```python
from build123d import *

# Parameters (mm, degrees)
EXTRUDE_1_DEPTH     = 8
SKETCH_3_R          = 16.5
CUT_EXTRUDE_1_DEPTH = 8
SKETCH_2_R          = 4
CUT_EXTRUDE_2_DEPTH = 60
SKETCH_4_R          = 4
CUT_EXTRUDE_3_DEPTH = 60
SKETCH_5_R          = 4
CUT_EXTRUDE_4_DEPTH = 60
SKETCH_6_R          = 4
CUT_EXTRUDE_5_DEPTH = 60
CUT_EXTRUDE_6_DEPTH = 1
SKETCH_8_R          = 2
CUT_EXTRUDE_8_DEPTH = 9


with BuildPart() as part:
    # 草图1 → 凸台-拉伸1 (new body)
    with BuildSketch(Plane(origin=(0, 0, 0), x_dir=(1, 0, 0), z_dir=(0, 1, 0))):
        Polygon((-40, 55), (-50, 45), (-50, -45), (-40, -55), (40, -55), (50, -45), (50, 45), (40, 55), align=None)
    extrude(amount=EXTRUDE_1_DEPTH)

    # 草图3 → 切除-拉伸1 (cut)
    with BuildSketch(Plane(origin=(0, 8, 0), x_dir=(1, 0, 0), z_dir=(0, 1, 0))):
        with Locations(Location((0, 0, 0), (0, 0, 270))):
            Circle(SKETCH_3_R)
    extrude(amount=-CUT_EXTRUDE_1_DEPTH, mode=Mode.SUBTRACT)

    # 草图2 → 切除-拉伸2 (cut)
    with BuildSketch(Plane(origin=(47.5, 0, 47.5), x_dir=(0.7071067811865483, 0, -0.7071067811865468), z_dir=(0.7071067811865468, 0, 0.7071067811865483))):
        with Locations((-3.535533906, 6)):
            Circle(SKETCH_2_R)
    extrude(amount=-CUT_EXTRUDE_2_DEPTH, mode=Mode.SUBTRACT)

    # 草图4 → 切除-拉伸3 (cut)
    with BuildSketch(Plane(origin=(-47.5, 0, 47.5), x_dir=(0.7071067811865475, 0, 0.7071067811865477), z_dir=(-0.7071067811865477, 0, 0.7071067811865475))):
        with Locations((3.535533906, 6)):
            Circle(SKETCH_4_R)
    extrude(amount=-CUT_EXTRUDE_3_DEPTH, mode=Mode.SUBTRACT)

    # 草图5 → 切除-拉伸4 (cut)
    with BuildSketch(Plane(origin=(-47.5, 0, -47.5), x_dir=(-0.7071067811865477, 0, 0.7071067811865475), z_dir=(-0.7071067811865475, 0, -0.7071067811865477))):
        with Locations((-3.535533906, 6)):
            Circle(SKETCH_5_R)
    extrude(amount=-CUT_EXTRUDE_4_DEPTH, mode=Mode.SUBTRACT)

    # 草图6 → 切除-拉伸5 (cut)
    with BuildSketch(Plane(origin=(47.5, 0, -47.5), x_dir=(-0.7071067811865475, 0, -0.7071067811865477), z_dir=(0.7071067811865477, 0, -0.7071067811865475))):
        with Locations((3.535533906, 6)):
            Circle(SKETCH_6_R)
    extrude(amount=-CUT_EXTRUDE_5_DEPTH, mode=Mode.SUBTRACT)

    # 草图7 → 切除-拉伸6 (cut)
    with BuildSketch(Plane(origin=(0, 8, 0), x_dir=(1, 0, 0), z_dir=(0, 1, 0))):
        Polygon((0, 47.334494774), (-7.385524007, 39.948970766), (7.385524007, 39.948970766), align=None)
    extrude(amount=-CUT_EXTRUDE_6_DEPTH, mode=Mode.SUBTRACT)

    # 草图8 → 切除-拉伸8 (cut)
    with BuildSketch(Plane(origin=(0, 8, 0), x_dir=(1, 0, 0), z_dir=(0, 1, 0))):
        with Locations(Location((-32.511046196, 47.511046196, 0), (0, 0, 270))):
            Circle(SKETCH_8_R)
        with Locations(Location((-42.504921706, 37.504921706, 0), (0, 0, 270))):
            Circle(SKETCH_8_R)
        with Locations(Location((-16.594623736, 31.594623736, 0), (0, 0, 270))):
            Circle(SKETCH_8_R)
        with Locations(Location((-26.594623736, 21.594623736, 0), (0, 0, 270))):
            Circle(SKETCH_8_R)
        with Locations(Location((16.828543077, 31.828543077, 0), (0, 0, 270))):
            Circle(SKETCH_8_R)
        with Locations(Location((32.511046196, 47.511046196, 0), (0, 0, 270))):
            Circle(SKETCH_8_R)
        with Locations(Location((42.504921706, 37.504921706, 0), (0, 0, 270))):
            Circle(SKETCH_8_R)
        with Locations(Location((26.57676385, 21.57676385, 0), (0, 0, 270))):
            Circle(SKETCH_8_R)
        with Locations(Location((-26.63034351, -21.63034351, 0), (0, 0, 270))):
            Circle(SKETCH_8_R)
        with Locations(Location((-16.8946096, -31.8946096, 0), (0, 0, 270))):
            Circle(SKETCH_8_R)
        with Locations(Location((-42.504921706, -37.504921706, 0), (0, 0, 270))):
            Circle(SKETCH_8_R)
        with Locations(Location((-32.684358037, -47.684358037, 0), (0, 0, 270))):
            Circle(SKETCH_8_R)
        with Locations(Location((26.558903963, -21.558903963, 0), (0, 0, 270))):
            Circle(SKETCH_8_R)
        with Locations(Location((17.062462418, -32.062462418, 0), (0, 0, 270))):
            Circle(SKETCH_8_R)
        with Locations(Location((42.504921706, -37.504921706, 0), (0, 0, 270))):
            Circle(SKETCH_8_R)
        with Locations(Location((32.355177206, -47.355177206, 0), (0, 0, 270))):
            Circle(SKETCH_8_R)
    extrude(amount=-CUT_EXTRUDE_8_DEPTH, mode=Mode.SUBTRACT)


solid = part.part
```
Work out the finished part from the listing and answer in its coordinate system (mm). A direction names the side the tool comes from. Coordinates: 2 decimals unless noted, no trailing zeros. Loops run counter-clockwise (first coordinate to the right, second up) from the corner with the lowest first, then second, coordinate; pieces in that order, holes last.
1) Section B-B (y = 5) is taken. Give the number of separate pieces and of enclosed holes in the cut face, plus the area to 3 significant figures.
Results:
separate pieces: 4
enclosed holes: 16
area: 8,160 mm2
2) Section A-A (z = 0) is taken. Give the vertices of the cut face in (x, y), plus the area to 3 significant figures.
Results:
outline: (-50, 0) - (-16.5, 0) - (-16.5, 8) - (-50, 8) - close; (16.5, 0) - (50, 0) - (50, 8) - (16.5, 8) - close
area: 536 mm2
3) For a pull along Y with two mould halves and no side action, classify faces 1 (the cylindrical face through (27, 2, 32)), 2 (the flat face through (3.744, 7.507, -43.59)), 3 (the flat face through (-1, 8, -36)) as +Y half, -Y half, draft (parallel to the pull), parting line (faces both ways), or undercut.
Results:
face 1: undercut
face 2: draft
face 3: +Y half
4) Consider probe 1 along Z at (x, y) = (30, 6); probe 2 along Z at (x, y) = (-42, 5.5); probe 3 along Z at (x, y) = (-22, 4). Determine where each line is inside the solid, lowest interval first.
Results:
probe 1: z = -55 to -40.66, -29.34 to 29.34, 40.66 to 55
probe 2: z = -53 to -52.61, -41.39 to -39.44, -35.57 to 35.57, 39.44 to 41.39, 52.61 to 53
probe 3: z = -55 to -31.9, -22.1 to 22.1, 31.9 to 55
5) For faces 4 (the flat face through (-3.641, 7.507, -43.693)), 5 (the flat face through (-46, 2, -49)), determine the directions among +Z, -Z, +X, -X, +Y, -Y from which every point of the face is accessible in a straight line to the end or side of a thin tool.
Results:
face 4: +Y
face 5: -Z, -X, +Y, -Y
6) A flat-ended cylindrical pin translates along its axis: pin 1 (3 mm diameter, centred on x = 42.5, z = -37.5, fed in from -Y). Find the tip coordinate at first contact, or state that the pin passes through.
Results:
pin 1: passes through
